```python
from build123d import *

# Parameters (mm, degrees)
ESBO_O1_W                                            = 42.10000000000001
ESBO_O1_H                                            = 42.10000000000002
RESSALTO_EXTRUS_O1_DEPTH                             = 4
ESBO_O2_R                                            = 12.000000000000007
CORTE_EXTRUS_O1_DEPTH                                = 8
ESCAREADO_PARA_PARAFUSO_DE_M_QUINA_COM_C_D           = 3.2
ESCAREADO_PARA_PARAFUSO_DE_M_QUINA_COM_C_CSINK_D     = 6.3
ESCAREADO_PARA_PARAFUSO_DE_M_QUINA_COM_C_CSINK_ANGLE = 90
RESSALTO_EXTRUS_O2_DEPTH                             = 10
ESBO_O6_R                                            = 3.5000000000000075
CORTE_EXTRUS_O2_DEPTH                                = 10.000000000000002
FURO_COM_FOLGA_DE_M31_D                              = 3.2
FILETE1_R                                            = 5
CORTE_EXTRUS_O6_DEPTH                                = 22.500000000000007
CHANFRO1_SIZE                                        = 2.7
SKETCH2_W                                            = 42.10000000000001
SKETCH2_H                                            = 14.000000000000002
SKETCH2_R                                            = 1.5999999999999908
BOSS_EXTRUDE1_DEPTH                                  = 1
RESSALTO_EXTRUS_O3_DEPTH                             = 5
FILETE3_R                                            = 10
ESBO_O17_R                                           = 1.5999999999999908
ESBO_O17_R_2                                         = 1.599999999999991
CORTE_EXTRUS_O8_DEPTH                                = 31
CORTE_EXTRUS_O9_DEPTH                                = 8
CORTE_EXTRUS_O9_DEPTH_BACK                           = 2


with BuildPart() as part:
    # Esboço1 → Ressalto-extrusão1 (new body)
    with BuildSketch(Plane.XY):
        with Locations((87.32270610713223, -330.71568115646056)):
            Rectangle(ESBO_O1_W, ESBO_O1_H)
    extrude(amount=RESSALTO_EXTRUS_O1_DEPTH)

    # Esboço2 → Corte-extrusão1 (cut)
    with BuildSketch(Plane.XY.offset(4)):
        with Locations((87.32270610713225, -330.71568115646056)):
            Circle(ESBO_O2_R)
    extrude(amount=-CORTE_EXTRUS_O1_DEPTH, mode=Mode.SUBTRACT)

    # Escareado para parafuso de máquina com cabeça chata de M31 (through all)
    with Locations(Plane.XY.offset(4)):
        with Locations((102.822706107, -346.215681156), (102.822706107, -315.215681156), (71.822706107, -315.215681156), (71.822706107, -346.215681156)):
            CounterSinkHole(ESCAREADO_PARA_PARAFUSO_DE_M_QUINA_COM_C_D / 2, ESCAREADO_PARA_PARAFUSO_DE_M_QUINA_COM_C_CSINK_D / 2, counter_sink_angle=ESCAREADO_PARA_PARAFUSO_DE_M_QUINA_COM_C_CSINK_ANGLE)

    # Esboço5 → Ressalto-extrusão2 (add)
    with BuildSketch(Plane.XY.offset(4)):
        with BuildLine():
            Line((99.98357100649832, -333.66568115646055), (108.37270610713225, -333.66568115646055))
            Line((108.37270610713225, -333.66568115646055), (108.37270610713225, -309.66568115646055))
            Line((108.37270610713225, -309.66568115646055), (66.27270610713224, -309.66568115646055))
            Line((66.27270610713224, -309.66568115646055), (66.27270610713224, -333.66568115646055))
            Line((66.27270610713224, -333.66568115646055), (74.66184120776617, -333.66568115646055))
            ThreePointArc((74.66184120776617, -333.66568115646055), (87.32270610713225, -317.71568115646056), (99.98357100649832, -333.66568115646055))
        make_face()
    extrude(amount=RESSALTO_EXTRUS_O2_DEPTH)

    # Esboço6 → Corte-extrusão2 (cut)
    with BuildSketch(Plane.XY.offset(14)):
        with Locations((71.82270610713223, -315.21568115646056)):
            Circle(ESBO_O6_R)
        with Locations((102.82270610713226, -315.21568115646056)):
            Circle(ESBO_O6_R)
    extrude(amount=-CORTE_EXTRUS_O2_DEPTH, mode=Mode.SUBTRACT)

    # Furo com folga de M31 (through all)
    with Locations(Plane(origin=(0, -309.66568115646055, 0), x_dir=(1, 0, 0), z_dir=(0, 1, 0))):
        with Locations((103.359135837, -8.012655369), (71.286276377, -8.012655369)):
            Hole(FURO_COM_FOLGA_DE_M31_D / 2)

    # Filete1
    # the kernel refuses this fillet: 5 mm, written as the material it adds along each edge
    with BuildSketch(Plane(origin=(87.48357100649832, -333.66568115646055, 4), x_dir=(0, -1, 0), z_dir=(1, 0, 0))) as filete1_piece_1_section:
        with BuildLine():
            CenterArc((FILETE1_R, -FILETE1_R), FILETE1_R, 90, 90)
            Line((0, -FILETE1_R), (0, 0))
            Line((0, 0), (FILETE1_R, 0))
        make_face()
    filete1_piece_1 = extrude(amount=20.889135100633922, mode=Mode.PRIVATE)
    filete1_piece_1 = filete1_piece_1 - Plane(origin=(87.32270610713225, -330.71568115646056, 5.015859225762799), x_dir=(-0.9739126845666216, -0.22692307692307614, 0), z_dir=(0, 0, -1)) * Cylinder(12.999999999999995, 62, mode=Mode.PRIVATE)
    filete1_piece_1 = filete1_piece_1 - Plane(origin=(103.359135837, -334.8905504329836, 8.012655369), x_dir=(-1, 0, 0), z_dir=(0, -1, 0)) * Cylinder(1.6, 62, mode=Mode.PRIVATE)
    add(filete1_piece_1)
    with BuildSketch(Plane(origin=(66.27270610713224, -333.66568115646055, 4), x_dir=(0, -1, 0), z_dir=(1, 0, 0))) as filete1_piece_2_section:
        with BuildLine():
            CenterArc((FILETE1_R, -FILETE1_R), FILETE1_R, 90, 90)
            Line((0, -FILETE1_R), (0, 0))
            Line((0, 0), (FILETE1_R, 0))
        make_face()
    filete1_piece_2 = extrude(amount=20.889135100633936, mode=Mode.PRIVATE)
    filete1_piece_2 = filete1_piece_2 - Plane(origin=(87.32270610713225, -330.71568115646056, 5.01585849038902), x_dir=(-0.9739126845666216, -0.22692307692307614, 0), z_dir=(0, 0, -1)) * Cylinder(12.999999999999995, 62, mode=Mode.PRIVATE)
    filete1_piece_2 = filete1_piece_2 - Plane(origin=(71.286276377, -334.8905494522985, 8.012655369), x_dir=(-1, 0, 0), z_dir=(0, -1, 0)) * Cylinder(1.6, 62, mode=Mode.PRIVATE)
    add(filete1_piece_2)
    # the kernel refuses this fillet: 5 mm, written as the material it takes off along each edge
    with BuildSketch(Plane(origin=(87.32270610713225, -330.71568115646056, 14), x_dir=(-0.36935058707522056, -0.9292901289840487, 0), z_dir=(0.9292901289840487, -0.36935058707522056, 0))) as filete1_2_piece_1:
        with BuildLine():
            CenterArc((12.999999999999979 + FILETE1_R, FILETE1_R), FILETE1_R, 180, 90)
            Line((12.999999999999979 + FILETE1_R, 0), (12.999999999999979, 0))
            Line((12.999999999999979, 0), (12.999999999999984, FILETE1_R))
        make_face()
    revolve(axis=Axis((87.32270610713225, -330.71568115646056, 14), (0, 0, -1)), revolution_arc=316.648856226302, mode=Mode.SUBTRACT)
    with BuildSketch(Plane(origin=(87.48357100649832, -333.66568115646055, 14), x_dir=(0, 0, -1), z_dir=(1, 0, 0))) as filete1_2_piece_2:
        with BuildLine():
            CenterArc((FILETE1_R, FILETE1_R), FILETE1_R, 180, 90)
            Line((0, FILETE1_R), (0, 0))
            Line((0, 0), (FILETE1_R, 0))
        make_face()
    extrude(amount=33.38913510063392, mode=Mode.SUBTRACT)
    with BuildSketch(Plane(origin=(53.77270610713224, -333.66568115646055, 14), x_dir=(0, 1, 0), z_dir=(1, 0, 0))) as filete1_2_piece_3:
        with BuildLine():
            CenterArc((FILETE1_R, -FILETE1_R), FILETE1_R, 90, 90)
            Line((0, -FILETE1_R), (0, 0))
            Line((0, 0), (FILETE1_R, 0))
        make_face()
    extrude(amount=33.389135100633936, mode=Mode.SUBTRACT)

    # Esboço13 → Corte-extrusão6 (cut)
    with BuildSketch(Plane.XZ.offset(351.7656811564606)):
        Polygon((74.0362763774125, 9.60036860941331), (71.28627637741243, 11.188081849684735), (68.53627637741243, 9.600368609413174), (68.53627637741253, 6.424942128870199), (71.2862763774126, 4.837228888598795), (74.03627637741259, 6.424942128870374), align=None)
        Polygon((106.10913583685199, 9.600368609413255), (103.35913583685196, 11.188081849684727), (100.60913583685196, 9.600368609413236), (100.60913583685199, 6.424942128870286), (103.359135836852, 4.837228888598834), (106.109135836852, 6.424942128870341), align=None)
    extrude(amount=-CORTE_EXTRUS_O6_DEPTH, mode=Mode.SUBTRACT)

    # Chanfro1
    chanfro1_edges = [part.edges().sort_by_distance(p)[0] for p in [
        (66.27270610713224, -351.7656811564606, 2),
        (108.37270610713225, -351.7656811564606, 2),
    ]]
    chamfer(chanfro1_edges, length=CHANFRO1_SIZE)

    # Sketch2 → Boss-Extrude1 (add)
    with BuildSketch(Plane(origin=(0, -309.66568115646055, 0), x_dir=(1, 0, 0), z_dir=(0, 1, 0))):
        with Locations((87.32270610713223, -7.000000000000001)):
            Rectangle(SKETCH2_W, SKETCH2_H)
        with Locations(Location((71.2862763774125, -8.012655369141836, 0), (0, 0, 270))):
            Circle(SKETCH2_R, mode=Mode.SUBTRACT)
        with Locations(Location((103.35913583685199, -8.012655369141836, 0), (0, 0, 270))):
            Circle(SKETCH2_R, mode=Mode.SUBTRACT)
    extrude(amount=BOSS_EXTRUDE1_DEPTH)

    # Esboço16 → Ressalto-extrusão3 (add)
    with BuildSketch(Plane.XZ.offset(308.6656811564605)):
        with BuildLine():
            Line((66.27270610713242, 0), (48.26899269713348, -2.2e-16))
            Line((48.26899269713348, -2.2e-16), (48.26899269713353, 9.000000000000064))
            ThreePointArc((48.26899269713353, 9.000000000000064), (49.147672353573896, 11.121320343559699), (51.268992697133534, 12.000000000000052))
            Line((51.268992697133534, 12.000000000000052), (60.2689926971336, 12.000000000000052))
            ThreePointArc((60.2689926971336, 12.000000000000052), (62.00104350470245, 12.550510257216857), (63.097419821879775, 14))
            Line((63.097419821879775, 14), (66.27270610713242, 14))
            Line((66.27270610713242, 14), (66.27270610713242, 0))
        make_face()
    extrude(amount=RESSALTO_EXTRUS_O3_DEPTH)

    # Filete3
    filete3_edges = [part.edges().sort_by_distance(p)[0] for p in [
        (66.27270610713227, -313.66568115646055, 7),
    ]]
    fillet(filete3_edges, radius=FILETE3_R)

    # Esboço17 → Corte-extrusão8 (cut)
    with BuildSketch(Plane(origin=(0, -308.66568115646055, 0), x_dir=(1, 0, 0), z_dir=(0, 1, 0))):
        with Locations(Location((83.76899269713277, -3.499999999999323, 0), (0, 0, 270))):
            Circle(ESBO_O17_R)
        with Locations(Location((52.76899269713277, -3.499999999999323, 0), (0, 0, 270))):
            Circle(ESBO_O17_R_2)
    extrude(amount=-CORTE_EXTRUS_O8_DEPTH, mode=Mode.SUBTRACT)

    # Esboço18 → Corte-extrusão9 (cut, two sides: drawn at the far end of the back side and taken through both)
    with BuildSketch(Plane.XZ.offset(313.6656811564605).offset(-CORTE_EXTRUS_O9_DEPTH_BACK)):
        Polygon((52.76899269713293, 6.674999999999326), (50.01936204011733, 5.087499999999323), (50.01936204011733, 1.9124999999993277), (52.76899269713293, 0.3249999999993254), (55.51862335414852, 1.9124999999993266), (55.51862335414852, 5.087499999999325), align=None)
        Polygon((83.76899269713292, 6.6749999999993275), (81.01936204011734, 5.087499999999328), (81.01936204011734, 1.9124999999993286), (83.76899269713293, 0.3249999999993267), (86.5186233541485, 1.9124999999993186), (86.5186233541485, 5.087499999999332), align=None)
    extrude(amount=CORTE_EXTRUS_O9_DEPTH + CORTE_EXTRUS_O9_DEPTH_BACK, mode=Mode.SUBTRACT)


solid = part.part
```
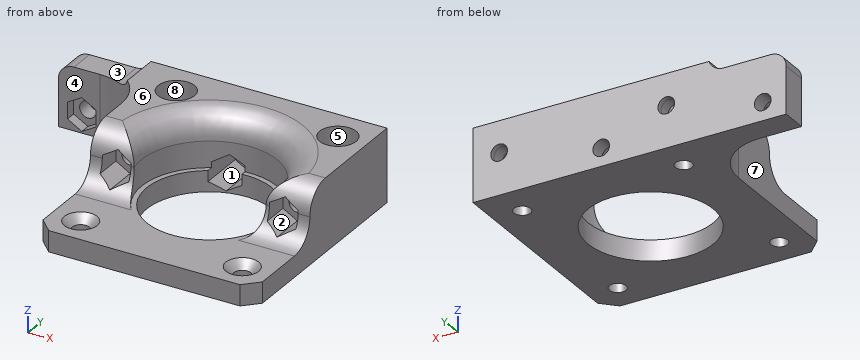
Design review of the part built by this model. Coordinates are the model's own, in mm. Face numbers are marked on the shaded views. A direction names the side the tool comes from. Give positions to 0.01 mm unless a question says otherwise; leave off trailing zeros. Use a Markdown table: item, result. Add a question column.
(1) Clearance check with flat-ended pins moving along their axes: P1, Ø3, axis at x = 103.5, z = 7, coming from the -Y side; P2, Ø3.5, axis at x = 103.36, z = 8.01, coming from the +Y side; P3, Ø2.5, axis at x = 71.29, z = 8.01, coming from the +Y side; P4, Ø8, axis at x = 94, y = -337.5, coming from the +Z side. State where each tip first meets the part, or that it passes through.
(2) Machinability: for the marked faces 1, 2, 3, 4 and 5, which of the approach directions +Z, -Z, +X, -X, +Y, -Y give a long, thin tool a straight path to every point of the face, cutting with its end or side? Answer none if there is none.
(3) Wall thickness on probe 1 along X at (y, z) = (-324, 7.75); probe 2 along Z at (x, y) = (59.5, -312); probe 3 along X at (y, z) = (-334, 6.75): over which ranges is each line inside the solid? List them lowest first. Write a range as [from, to].
(4) Mouldability with a two-part tool opening along X and no side actions: class the marked faces 6, 7 and 8 as +X half, -X half, draft (parallel to the pull), parting line (faces both ways), or undercut.
Report:
| question | item | result |
|---|---|---|
| 1 | P1 | stops at y = -329.27 |
| 1 | P2 | stops at y = -308.67 |
| 1 | P3 | passes through |
| 1 | P4 | stops at z = 4.02 |
| 2 | face 1 | none |
| 2 | face 2 | -Y |
| 2 | face 3 | +Z, -X, +Y, -Y |
| 2 | face 4 | +Z, -Z, -X, -Y |
| 2 | face 5 | +Z |
| 3 | probe 1 | x = [66.27, 69.71], [72.86, 76.19], [98.45, 101.78], [104.94, 108.37] |
| 3 | probe 2 | z = [0, 12] |
| 3 | probe 3 | x = [66.27, 68.54], [74.04, 74.74], [99.9, 100.61], [106.11, 108.37] |
| 4 | face 6 | draft |
| 4 | face 7 | -X half |
| 4 | face 8 | undercut |
